Build history of the part. All positions in model axes, mm. Give positions to 0.01 mm unless a question says otherwise; leave off trailing zeros. Write each loop counter-clockwise with the first axis right and the second up, starting at its lowest first coordinate (ties: lowest second). Pieces come first, ordered by that corner, then holes. Notation, with made-up numbers: (43.5, -31) -> (84.5, -31) arc R9 cw to (84.5, -15) -> close; hole circle Ø5 at (65, 65.25). An arc over 180 degrees is marked (long way). Put each result on its own line as item: value.
from build123d import *

# Parameters (mm, degrees)
SKETCH1_W           = 279.4
SKETCH1_H           = 133.35
BOSS_EXTRUDE1_DEPTH = 1.3335
CUT_EXTRUDE2_START  = 1.3335
SKETCH2_R           = 38.8874
CUT_EXTRUDE2_DEPTH  = 157.134739812
CUT_EXTRUDE4_START  = 1.3335
SKETCH3_R           = 2.7686
CUT_EXTRUDE4_DEPTH  = 157.134739812


with BuildPart() as part:
    # Sketch1 → Boss-Extrude1 (new, symmetric)
    with BuildSketch(Plane(origin=(0, 0, 0), x_dir=(1, 0, 0), z_dir=(0, 1, 0))):
        Rectangle(SKETCH1_W, SKETCH1_H)
    extrude(amount=BOSS_EXTRUDE1_DEPTH, both=True)

    # Sketch2 → Cut-Extrude2 (cut, through all)
    with BuildSketch(Plane(origin=(0, 0, 0), x_dir=(1, 0, 0), z_dir=(0, 1, 0)).offset(CUT_EXTRUDE2_START)):
        with Locations((0, 66.675)):
            Circle(SKETCH2_R)
    extrude(amount=-CUT_EXTRUDE2_DEPTH, mode=Mode.SUBTRACT)

    # Sketch3 → Cut-Extrude4 (cut, through all)
    with BuildSketch(Plane(origin=(0, 0, 0), x_dir=(1, 0, 0), z_dir=(0, 1, 0)).offset(CUT_EXTRUDE4_START)):
        with Locations(Location((-133.35, -57.15, 0), (0, 0, 270))):
            Circle(SKETCH3_R)
        with Locations(Location((133.35, -57.15, 0), (0, 0, 270))):
            Circle(SKETCH3_R)
        with Locations(Location((-133.35, 57.15, 0), (0, 0, 270))):
            Circle(SKETCH3_R)
        with Locations(Location((133.35, 57.15, 0), (0, 0, 270))):
            Circle(SKETCH3_R)
    extrude(amount=-CUT_EXTRUDE4_DEPTH, mode=Mode.SUBTRACT)


solid = part.part
1) Wall check: L1, parallel to Z at x = 133.35, y = -0.45 (3 decimals); L2, parallel to X at y = 0.2, z = 57.15; L3, parallel to X at y = 0.75, z = -57.15. Give the ranges that are in metal, low to high.
Filled sheet:
L1: -66.675 to -59.919, -54.381 to 54.381, 59.919 to 66.675
L2: -139.7 to -136.12, -130.58 to 130.58, 136.12 to 139.7
L3: -139.7 to -136.12, -130.58 to -37.7, 37.7 to 130.58, 136.12 to 139.7
2) Slice it at A-A (z = 57.15). Write the cut outline in (x, y).
Filled sheet:
outline: (-139.7, -1.33) -> (-136.12, -1.33) -> (-136.12, 1.33) -> (-139.7, 1.33) -> close; (-130.58, -1.33) -> (130.58, -1.33) -> (130.58, 1.33) -> (-130.58, 1.33) -> close; (136.12, -1.33) -> (139.7, -1.33) -> (139.7, 1.33) -> (136.12, 1.33) -> close
3) Slice it at B-B (y = 0.5). Write the cut outline in (x, z) (3 decimals), plus the area to 3 significant figures.
Filled sheet:
outline: (-139.7, -66.675) -> (-38.887, -66.675) arc R38.887 cw to (38.887, -66.675) -> (139.7, -66.675) -> (139.7, 66.675) -> (-139.7, 66.675) -> close; hole circle Ø5.537 at (-133.35, -57.15); hole circle Ø5.537 at (-133.35, 57.15); hole circle Ø5.537 at (133.35, -57.15); hole circle Ø5.537 at (133.35, 57.15)
area: 34,800 mm2
4) Pull direction Z, two halves, no side cores. Call faces 1 (the cylindrical face through (-0.9, 0, -27.8)), 2 (the flat face through (-2, 1.334, -1)), 3 (the cylindrical face through (-130.605, 0.019, 56.79)): released by +Z, released by -Z, zero draft, split by the parting line, or undercut.
Filled sheet:
face 1: released by -Z
face 2: zero draft
face 3: undercut
5) Slice it at C-C (x = 133.35). Write the cut outline in (y, z) (1 decimal).
Filled sheet:
outline: (-1.3, -66.7) -> (1.3, -66.7) -> (1.3, -59.9) -> (-1.3, -59.9) -> close; (-1.3, -54.4) -> (1.3, -54.4) -> (1.3, 54.4) -> (-1.3, 54.4) -> close; (-1.3, 59.9) -> (1.3, 59.9) -> (1.3, 66.7) -> (-1.3, 66.7) -> close
6) Slice it at D-D (z = -57.15). Write the cut outline in (x, y).
Filled sheet:
outline: (-139.7, -1.33) -> (-136.12, -1.33) -> (-136.12, 1.33) -> (-139.7, 1.33) -> close; (-130.58, -1.33) -> (-37.7, -1.33) -> (-37.7, 1.33) -> (-130.58, 1.33) -> close; (37.7, -1.33) -> (130.58, -1.33) -> (130.58, 1.33) -> (37.7, 1.33) -> close; (136.12, -1.33) -> (139.7, -1.33) -> (139.7, 1.33) -> (136.12, 1.33) -> close
